```python
from build123d import *

# Parameters (mm, degrees)
PAD_DEPTH       = 45
SKETCH001_R     = 2
SKETCH001_R_2   = 2.35
SKETCH001_W     = 3
SKETCH001_H     = 5
SKETCH001_W_2   = 5
SKETCH001_H_2   = 15
POCKET_DEPTH    = 45.001
SKETCH002_W     = 45
SKETCH002_H     = 32.5
POCKET001_DEPTH = 74.001
POCKET002_DEPTH = 33
SKETCH004_R     = 2.35
POCKET003_DEPTH = 9
SKETCH005_W     = 47.5
SKETCH005_H     = 20
POCKET004_DEPTH = 4
POCKET005_DEPTH = 30
SKETCH007_W     = 19
SKETCH007_H     = 4
POCKET006_DEPTH = 3
POCKET007_DEPTH = 4
POCKET008_DEPTH = 55.751
POCKET009_DEPTH = 15
PAD001_DEPTH    = 9
POCKET010_DEPTH = 45.001
SKETCH013_R     = 2.75
POCKET011_DEPTH = 0.75
SKETCH014_R     = 2.75
POCKET012_DEPTH = 0.75
SKETCH015_W     = 24
SKETCH015_H     = 12.5
PAD002_DEPTH    = 2
POCKET013_DEPTH = 74.001
CHAMFER_SIZE    = 2
FILLET_R        = 4
CHAMFER001_SIZE = 1.5
CHAMFER002_SIZE = 1
FILLET001_R     = 3
FILLET002_R     = 5
FILLET003_R     = 3.99
FILLET004_R     = 4
POCKET014_DEPTH = 55.751
POCKET015_DEPTH = 2
CHAMFER003_SIZE = 1.49
SKETCH019_W     = 5
SKETCH019_H     = 8
POCKET016_DEPTH = 7


with BuildPart() as part:
    # Sketch → Pad (new body)
    with BuildSketch(Plane.XY):
        Polygon((74, -15.75), (74, 0), (0, 0), (0, -15.75), (24, -15.75), (24, -55.75), (50, -55.75), (50, -15.75), align=None)
    extrude(amount=PAD_DEPTH)

    # Sketch001 (on Face9 of Pad) → Pocket (cut, through all)
    with BuildSketch(Plane(origin=(0, 0, 0), x_dir=(1, 0, 0), z_dir=(0, 0, -1))):
        with Locations((36.5, 43.25)):
            Circle(SKETCH001_R)
        with Locations((37, 51)):
            Circle(SKETCH001_R_2)
        with Locations((43.25, 51)):
            Rectangle(SKETCH001_W, SKETCH001_H)
        Polygon((0, 8), (8, 0), (0, 0), align=None)
        with Locations((66, 7.5)):
            Rectangle(SKETCH001_W_2, SKETCH001_H_2)
    extrude(amount=-POCKET_DEPTH, mode=Mode.SUBTRACT)

    # Sketch002 (on Face1 of Pocket) → Pocket001 (cut, through all)
    with BuildSketch(Plane.YZ.offset(74)):
        with Locations((-38.25, 28.75)):
            Rectangle(SKETCH002_W, SKETCH002_H)
    extrude(amount=-POCKET001_DEPTH, mode=Mode.SUBTRACT)

    # Sketch003 (on Face4 of Pocket001) → Pocket002 (cut)
    with BuildSketch(Plane.XY.offset(45)):
        Polygon((45.75, -15.75), (49.9375, -11.5625), (58.5625, -11.5625), (62.75, -15.75), align=None)
    extrude(amount=-POCKET002_DEPTH, mode=Mode.SUBTRACT)

    # Sketch004 (on Face15 of Pocket002) → Pocket003 (cut)
    with BuildSketch(Plane(origin=(0, 0, 0), x_dir=(-1, 0, 0), z_dir=(0, 1, 0))):
        with Locations((-57, 21)):
            Circle(SKETCH004_R)
        with Locations((-17, 21)):
            Circle(SKETCH004_R)
        Polygon((-43.25, 45), (-53.25, 35), (-53.25, 0), (-20.75, 0), (-20.75, 35), (-30.75, 45), align=None)
    extrude(amount=-POCKET003_DEPTH, mode=Mode.SUBTRACT)

    # Sketch005 (on Face19 of Pocket003) → Pocket004 (cut)
    with BuildSketch(Plane(origin=(0, 0, 0), x_dir=(-1, 0, 0), z_dir=(0, 1, 0))):
        with Locations((-37, 35)):
            Rectangle(SKETCH005_W, SKETCH005_H)
    extrude(amount=-POCKET004_DEPTH, mode=Mode.SUBTRACT)

    # Sketch006 (on Face17 of Pocket004) → Pocket005 (cut)
    with BuildSketch(Plane(origin=(0, -9, 0), x_dir=(-1, 0, 0), z_dir=(0, 1, 0))):
        with BuildLine():
            ThreePointArc((-32.5, 4), (-37, 8.5), (-41.5, 4))
            Line((-41.5, 4), (-41.5, 0))
            ThreePointArc((-41.5, 0), (-37, -4.5), (-32.5, 0))
            Line((-32.5, 4), (-32.5, 0))
        make_face()
    extrude(amount=-POCKET005_DEPTH, mode=Mode.SUBTRACT)

    # Sketch007 (on Face4 of Pocket005) → Pocket006 (cut)
    with BuildSketch(Plane(origin=(0, 0, 0), x_dir=(1, 0, 0), z_dir=(0, 0, -1))):
        with Locations((37, 29.5)):
            Rectangle(SKETCH007_W, SKETCH007_H)
    extrude(amount=-POCKET006_DEPTH, mode=Mode.SUBTRACT)

    # Sketch008 (on Face23 of Pocket006) → Pocket007 (cut)
    with BuildSketch(Plane(origin=(0, -31.5, 0), x_dir=(-1, 0, 0), z_dir=(0, 1, 0))):
        Polygon((-43.5, 3), (-43.5, 10), (-30.5, 10), (-30.5, 3), (-27.5, 3), (-27.5, 12.5), (-46.5, 12.5), (-46.5, 3), align=None)
    extrude(amount=POCKET007_DEPTH, mode=Mode.SUBTRACT)

    # Sketch009 (on Face14 of Pocket007) → Pocket008 (cut, through all)
    with BuildSketch(Plane(origin=(0, 0, 0), x_dir=(-1, 0, 0), z_dir=(0, 1, 0))):
        Polygon((0, 25), (-11, 14), (-11, 0), (0, 0), align=None)
    extrude(amount=-POCKET008_DEPTH, mode=Mode.SUBTRACT)

    # Sketch010 (on Face23 of Pocket008) → Pocket009 (cut)
    with BuildSketch(Plane(origin=(0, 0, 0), x_dir=(-1, 0, 0), z_dir=(0, 1, 0))):
        Polygon((-63.5, 39.25), (-62.25, 38), (-62.25, 27), (-63.5, 27), align=None)
    extrude(amount=-POCKET009_DEPTH, mode=Mode.SUBTRACT)

    # Sketch011 (on Face15 of Pocket009) → Pad001 (join)
    with BuildSketch(Plane.YZ.offset(32.5)):
        Polygon((-39, 0), (-39, 8.5), (-30.5, 8.5), align=None)
    extrude(amount=PAD001_DEPTH)

    # Sketch012 (on Face4 of Pad001) → Pocket010 (cut, through all)
    with BuildSketch(Plane(origin=(0, 0, 0), x_dir=(1, 0, 0), z_dir=(0, 0, -1))):
        with BuildLine():
            Line((30, 58), (33.25, 54.75))
            Line((33.25, 54.75), (37, 54.75))
            ThreePointArc((37, 54.75), (40.535534, 56.214466), (42, 59.75))
            Line((30, 59.75), (42, 59.75))
            Line((30, 58), (30, 59.75))
        make_face()
    extrude(amount=-POCKET010_DEPTH, mode=Mode.SUBTRACT)

    # Sketch013 (on Face4 of Pocket010) → Pocket011 (cut)
    with BuildSketch(Plane(origin=(0, 0, 0), x_dir=(1, 0, 0), z_dir=(0, 0, -1))):
        with Locations((37, 51)):
            Circle(SKETCH013_R)
    extrude(amount=-POCKET011_DEPTH, mode=Mode.SUBTRACT)

    # Sketch014 (on Face30 of Pocket011) → Pocket012 (cut)
    with BuildSketch(Plane(origin=(0, 0, 0), x_dir=(-1, 0, 0), z_dir=(0, 1, 0))):
        with Locations((-57, 21)):
            Circle(SKETCH014_R)
        with Locations((-17, 21)):
            Circle(SKETCH014_R)
    extrude(amount=-POCKET012_DEPTH, mode=Mode.SUBTRACT)

    # Sketch015 (on Face2 of Pocket012) → Pad002 (join)
    with BuildSketch(Plane.XZ.offset(15.75)):
        with Locations((62, 6.25)):
            Rectangle(SKETCH015_W, SKETCH015_H)
    extrude(amount=PAD002_DEPTH)

    # Sketch016 (on Face62 of Pad002) → Pocket013 (cut, through all)
    with BuildSketch(Plane.YZ.offset(74)):
        Polygon((-10, 0), (0, 10), (0, 0), align=None)
        Polygon((-5, 45), (0, 40), (0, 45), align=None)
        Polygon((-15.75, 40.75), (-10.25, 45), (-15.75, 45), align=None)
    extrude(amount=-POCKET013_DEPTH, mode=Mode.SUBTRACT)

    # Chamfer
    chamfer_edges = [part.edges().sort_by_distance(p)[0] for p in [
        (74, 0, 25),
        (74, -5, 5),
        (74, -2.5, 42.5),
    ]]
    chamfer(chamfer_edges, length=CHAMFER_SIZE)

    # Fillet
    fillet_edges = [part.edges().sort_by_distance(p)[0] for p in [
        (37, -9, 8.5),
    ]]
    fillet(fillet_edges, radius=FILLET_R)

    # Chamfer001
    chamfer001_edges = [part.edges().sort_by_distance(p)[0] for p in [
        (34.5, -43.25, 0),
    ]]
    chamfer(chamfer001_edges, length=CHAMFER001_SIZE)

    # Chamfer002
    chamfer002_edges = [part.edges().sort_by_distance(p)[0] for p in [
        (41.75, -51, 0),
        (43.25, -53.5, 0),
        (44.75, -51, 0),
        (43.25, -48.5, 0),
    ]]
    chamfer(chamfer002_edges, length=CHAMFER002_SIZE)

    # Fillet001
    fillet001_edges = [part.edges().sort_by_distance(p)[0] for p in [
        (43.5, -29.5, 10),
        (30.5, -29.5, 10),
    ]]
    fillet(fillet001_edges, radius=FILLET001_R)

    # Fillet002
    fillet002_edges = [part.edges().sort_by_distance(p)[0] for p in [
        (13.25, -2, 25),
        (60.75, -2, 25),
    ]]
    fillet(fillet002_edges, radius=FILLET002_R)

    # Fillet003
    fillet003_edges = [part.edges().sort_by_distance(p)[0] for p in [
        (13.25, -4, 37),
        (60.75, -4, 37),
    ]]
    fillet(fillet003_edges, radius=FILLET003_R)

    # Fillet004
    fillet004_edges = [part.edges().sort_by_distance(p)[0] for p in [
        (24, -55.75, 6.25),
        (50, -55.75, 6.25),
    ]]
    fillet(fillet004_edges, radius=FILLET004_R)

    # Sketch017 (on Face56 of Fillet004) → Pocket014 (cut, through all)
    with BuildSketch(Plane(origin=(0, 0, 0), x_dir=(-1, 0, 0), z_dir=(0, 1, 0))):
        with BuildLine():
            ThreePointArc((-30, 38.5), (-32, 40.5), (-34, 38.5))
            Line((-34, 38.5), (-34, 36.5))
            ThreePointArc((-34, 36.5), (-32, 34.5), (-30, 36.5))
            Line((-30, 38.5), (-30, 36.5))
        make_face()
    extrude(amount=-POCKET014_DEPTH, mode=Mode.SUBTRACT)

    # Sketch018 (on Face50 of Pocket014) → Pocket015 (cut)
    with BuildSketch(Plane(origin=(0, -9, 0), x_dir=(-1, 0, 0), z_dir=(0, 1, 0))):
        with BuildLine():
            ThreePointArc((-28.5, 38.5), (-32, 42), (-35.5, 38.5))
            Line((-35.5, 38.5), (-35.5, 36.5))
            ThreePointArc((-35.5, 36.5), (-32, 33), (-28.5, 36.5))
            Line((-28.5, 38.5), (-28.5, 36.5))
        make_face()
    extrude(amount=-POCKET015_DEPTH, mode=Mode.SUBTRACT)

    # Chamfer003
    chamfer003_edges = [part.edges().sort_by_distance(p)[0] for p in [
        (32, -11, 40.5),
    ]]
    chamfer(chamfer003_edges, length=CHAMFER003_SIZE)

    # Sketch019 (on Face10 of Chamfer003) → Pocket016 (cut)
    with BuildSketch(Plane.XY.offset(12.5)):
        with BuildLine():
            Line((26.5, -51.25), (26.5, -34.25))
            Line((26.5, -34.25), (47.5, -34.25))
            Line((47.5, -34.25), (47.5, -46.25))
            Line((47.5, -46.25), (40.5, -46.25))
            Line((40.5, -46.25), (40.5, -43.25))
            ThreePointArc((40.5, -43.25), (36.5, -39.25), (32.5, -43.25))
            Line((32.5, -43.25), (32.5, -51.25))
            Line((32.5, -51.25), (26.5, -51.25))
        make_face()
        with Locations((29, -21.25)):
            Rectangle(SKETCH019_W, SKETCH019_H)
        with Locations((45, -21.25)):
            Rectangle(SKETCH019_W, SKETCH019_H)
    extrude(amount=-POCKET016_DEPTH, mode=Mode.SUBTRACT)


solid = part.part
```
The listing builds one solid part. Answer for the finished solid, in the listing's coordinates (mm). A direction names the side the tool comes from. Give positions to 0.01 mm unless a question says otherwise; leave off trailing zeros. Write each loop counter-clockwise with the first axis right and the second up, starting at its lowest first coordinate (ties: lowest second). Pieces come first, ordered by that corner, then holes. Notation, with made-up numbers: (16.25, 83) -> (35.25, 83) arc R23 ccw to (35.25, 117) -> close; hole circle Ø6 at (53.25, 38.5). An arc over 180 degrees is marked (long way). Use one line per item in the form item = value.
1) Section C-C on x = 67 is taken. Write down the section's boundary in (y, z), plus the area to 3 significant figures.
Result:
outline = (-17.75, 0) -> (-15, 0) -> (-15, 41.33) -> (-15.75, 40.75) -> (-15.75, 12.5) -> (-17.75, 12.5) -> close
area = 55.8 mm²
2) A tool of negligible diameter and unlimited length cuts with its end or side. For faces 4 (the cylindrical face through (32, -14.1, 40.5)), 5 (the flat face through (42, -30, 3)), 6 (the flat face through (29, -21, 5.5)), 7 (the flat face through (53.25, -5, 18)), 8 (the cylindrical face through (54.52, -2.8, 26.14)), from which of +Z, -Z, +X, -X, +Y, -Y can it reach the whole face along a straight path? Write none if from no direction.
Result:
face_4 = +Y, -Y
face_5 = -Z
face_6 = +Z
face_7 = -Z, +Y
face_8 = +Z, +Y
3) Straight lines are drawn through the part: probe 1 along X at (y, z) = (-43.25, 7.75); probe 2 along X at (y, z) = (-4.5, 30.5); probe 3 along X at (y, z) = (-51, 0.25). For each, find the intervals that lie inside material, in ascending order.
Result:
probe_1 = 24 to 26.5, 32.5 to 34.5, 38.5 to 40.5, 47.5 to 50
probe_2 = 3.5 to 20.75, 53.25 to 62.25, 68.5 to 74
probe_3 = 24 to 34.25, 39.75 to 41, 45.5 to 50
4) Each of these flat-tipped pins is pushed along its axis until it touches: P1, Ø3.5, axis at y = -44.5, z = 10, coming from the +X side; P2, Ø14, axis at x = 58.5, z = 6, coming from the -Y side; P3, Ø12.5, axis at x = 68, z = 30.5, coming from the -Y side. Where does it stop, or does it pass through?
Result:
P1 = 50
P2 = -17.75
P3 = -15.75
5) For a pull along X with two mould halves and no side action, classify faces 1 (the flat face through (46.5, -29, 6)), 2 (the flat face through (7, -10, 18)), 3 (the flat face through (58, 0, 18)) as +X half, -X half, draft (parallel to the pull), parting line (faces both ways), or undercut.
Result:
face_1 = undercut
face_2 = -X half
face_3 = draft
6) Section D-D on z = 16 is taken. Write down the section's boundary in (x, y), plus the area to 3 significant figures.
Result:
outline = (9, -15.75) -> (45.75, -15.75) -> (49.94, -11.56) -> (58.56, -11.56) -> (62.75, -15.75) -> (74, -15.75) -> (74, -2) -> (72, 0) -> (68.5, 0) -> (68.5, -15) -> (63.5, -15) -> (63.5, 0) -> (53.25, 0) -> (53.25, -9) -> (20.75, -9) -> (20.75, 0) -> (9, 0) -> close
area = 601 mm²
7) Section B-B on y = -24 is taken. Write down the section's boundary in (x, z), plus the area to 3 significant figures.
Result:
outline = (24, 0) -> (32.5, 0) -> (32.5, 4) arc R4.5 cw to (41.5, 4) -> (41.5, 0) -> (50, 0) -> (50, 12.5) -> (47.5, 12.5) -> (47.5, 5.5) -> (42.5, 5.5) -> (42.5, 12.5) -> (31.5, 12.5) -> (31.5, 5.5) -> (26.5, 5.5) -> (26.5, 12.5) -> (24, 12.5) -> close
area = 187 mm²
